from build123d import *

# Parameters (mm, degrees)
SKETCH3_W               = 1.778
SKETCH3_H               = 21.844
SKETCH4_W               = 63.2968
SKETCH4_H               = 43.561
BOSS_EXTRUDE1_DEPTH     = 1.778
BOSS_EXTRUDE2_DEPTH     = 1.778
SKETCH6_R               = 1.8034
BOSS_EXTRUDE3_DEPTH     = 5.08
FILLET2_R               = 3.81
SKETCH7_R               = 1.8034
BOSS_EXTRUDE4_DEPTH     = 25.4
CUT_EXTRUDE1_DEPTH      = 82.893164904
CUT_EXTRUDE1_DEPTH_BACK = 82.893164904
SKETCH8_W               = 7.5438
SKETCH8_H               = 10.541
SKETCH13_R              = 2.52476
BOSS_EXTRUDE5_DEPTH     = 63.2968
SKETCH14_W              = 27.40279
SKETCH14_H              = 7.62
SKETCH14_H_2            = 8.382
SKETCH14_W_2            = 3.45694
CUT_EXTRUDE2_DEPTH      = 80.858589657
FILLET3_R               = 8.382
FILLET4_R               = 1.27


# Some blends are built 0.0001 mm under size
with BuildPart() as part:
    # Sweep1: sweep along a path in Sketch1
    with BuildLine(Plane.XY) as sweep1_path:
        Line((0, 41.783), (0, 0))
        Line((0, 0), (59.7408, 0))
        Line((59.7408, 0), (59.7408, 41.783))
    # Sketch3 → Sweep1 (sweep)
    with BuildSketch(Plane(origin=(0, 41.783, 0), x_dir=(1, 0, 0), z_dir=(0, 1, 0))):
        with Locations((-0.889, 0)):
            Rectangle(SKETCH3_W, SKETCH3_H)
    sweep(path=sweep1_path.line, transition=Transition.RIGHT)

    # Sketch4 → Boss-Extrude1 (add)
    with BuildSketch(Plane(origin=(0, 0, -10.922), x_dir=(-1, 0, 0), z_dir=(0, 0, -1))):
        with Locations((-29.8704, 20.0025)):
            Rectangle(SKETCH4_W, SKETCH4_H)
    extrude(amount=BOSS_EXTRUDE1_DEPTH)

    # Sketch5 → Boss-Extrude2 (add)
    # profile 1 of 2: a face of its own
    with BuildSketch(Plane.XY.offset(10.922)):
        with BuildLine():
            Line((30.2514, 41.783), (0, 41.783))
            Line((0, 41.783), (0, 0))
            Line((0, 0), (59.7408, 0))
            Line((59.7408, 0), (59.7408, 41.783))
            Line((59.7408, 41.783), (58.20156, 41.783))
            Line((58.20156, 41.783), (58.20156, 27.91968))
            ThreePointArc((58.20156, 27.91968), (44.22648, 13.9446), (30.2514, 27.91968))
            Line((30.2514, 27.91968), (30.2514, 41.783))
        make_face()
        with BuildLine():
            Line((4.445, 5.4864), (4.445, 34.798))
            ThreePointArc((4.445, 34.798), (5.188948776, 36.594051224), (6.985, 37.338))
            Line((6.985, 37.338), (18.6182, 37.338))
            ThreePointArc((18.6182, 37.338), (20.414251224, 36.594051224), (21.1582, 34.798))
            Line((21.1582, 34.798), (21.1582, 24.296354404))
            ThreePointArc((21.1582, 24.296354404), (21.641564969, 21.866314608), (23.018071939, 19.806226343))
            Line((23.018071939, 19.806226343), (25.343528061, 17.480770222))
            ThreePointArc((25.343528061, 17.480770222), (26.720035031, 15.420681957), (27.2034, 12.990642162))
            Line((27.2034, 12.990642162), (27.2034, 5.4864))
            ThreePointArc((27.2034, 5.4864), (26.459451224, 3.690348776), (24.6634, 2.9464))
            Line((24.6634, 2.9464), (6.985, 2.9464))
            ThreePointArc((6.985, 2.9464), (5.188948776, 3.690348776), (4.445, 5.4864))
        make_face(mode=Mode.SUBTRACT)
    # profile 2 of 2: a face of its own
    with BuildSketch(Plane.XY.offset(10.922)):
        Polygon((61.5188, 41.783), (59.7408, 41.783), (59.7408, 0), (0, 0), (0, 41.783), (-1.778, 41.783), (-1.778, -1.778), (61.5188, -1.778), align=None)
    extrude(amount=BOSS_EXTRUDE2_DEPTH)

    # Sketch6 → Boss-Extrude3 (add)
    with BuildSketch(Plane(origin=(0, 41.783, 0), x_dir=(1, 0, 0), z_dir=(0, 1, 0))):
        with BuildLine():
            Line((64.5922, 3.5814), (61.5188, 3.5814))
            Line((61.5188, 3.5814), (61.5188, -3.5814))
            Line((61.5188, -3.5814), (64.5922, -3.5814))
            ThreePointArc((64.5922, -3.5814), (68.1736, 0), (64.5922, 3.5814))
        make_face()
        with Locations(Location((64.5922, 0, 0), (0, 0, 180))):
            Circle(SKETCH6_R, mode=Mode.SUBTRACT)
    extrude(amount=-BOSS_EXTRUDE3_DEPTH)

    # Fillet2
    # the kernel refuses this fillet: 3.81 mm, written as the material it adds along each edge
    with BuildSketch(Plane(origin=(61.5188, 41.783, -3.5814), x_dir=(0, 0, -1), z_dir=(0, -1, 0))) as fillet2_piece_1:
        with BuildLine():
            CenterArc((3.773204979, 3.81), FILLET2_R, 185.719382358, 84.280617642)
            Line((-0.017828515, 3.430309278), (-0.396931865, 3.392340206))
            ThreePointArc((-0.396931865, 3.392340206), (-0.381, 3.0734), (-0.381, 0))
            Line((-0.381, 0), (0, -0.381))
            Line((0, -0.381), (3.773204979, -0.381))
            Line((3.773204979, -0.381), (3.773204979, 0))
        make_face()
    extrude(amount=5.08)
    with BuildSketch(Plane(origin=(61.5188, 41.783, 3.5814), x_dir=(0, 0, 1), z_dir=(0, -1, 0))) as fillet2_piece_2:
        with BuildLine():
            CenterArc((3.773204979, -3.81), FILLET2_R, 90, 84.280617642)
            Line((-0.017828515, -3.430309278), (-0.396931865, -3.392340206))
            ThreePointArc((-0.396931865, -3.392340206), (-0.381, -3.0734), (-0.381, 0))
            Line((-0.381, 0), (0, 0.381))
            Line((0, 0.381), (3.773204979, 0.381))
            Line((3.773204979, 0.381), (3.773204979, 0))
        make_face()
    extrude(amount=5.08)

    # Sketch7 → Boss-Extrude4 (add)
    with BuildSketch(Plane.XY.offset(12.7)):
        with BuildLine():
            Line((-1.778, 36.3982), (-1.778, 41.783))
            Line((-1.778, 41.783), (-3.902308892, 43.053335031))
            ThreePointArc((-3.902308892, 43.053335031), (-8.404920605, 42.372664125), (-8.599730754, 37.82306259))
            Line((-8.599730754, 37.82306259), (-1.778, 28.7782))
            Line((-1.778, 28.7782), (-1.778, 36.3982))
        make_face()
        with Locations((-5.7404, 39.9796)):
            Circle(SKETCH7_R, mode=Mode.SUBTRACT)
    extrude(amount=-BOSS_EXTRUDE4_DEPTH)

    # Sketch8 → Cut-Extrude1 (cut, two sides: drawn at the far end of the back side and taken through both)
    with BuildSketch(Plane(origin=(0, 41.783, 0), x_dir=(1, 0, 0), z_dir=(0, 1, 0)).offset(-CUT_EXTRUDE1_DEPTH_BACK)):
        with Locations((-5.5499, 7.4295)):
            Rectangle(SKETCH8_W, SKETCH8_H)
        with Locations((-5.5499, -7.4295)):
            Rectangle(SKETCH8_W, SKETCH8_H)
    extrude(amount=CUT_EXTRUDE1_DEPTH + CUT_EXTRUDE1_DEPTH_BACK, mode=Mode.SUBTRACT)

    # Sketch13 → Boss-Extrude5 (add)
    with BuildSketch(Plane.ZY.offset(1.778)):
        with BuildLine():
            Line((-21.082, -1.778), (-12.7, -1.778))
            Line((-12.7, -1.778), (-12.7, 13.462))
            Line((-12.7, 13.462), (-21.082, 13.462))
            ThreePointArc((-21.082, 13.462), (-28.702, 5.842), (-21.082, -1.778))
        make_face()
        with Locations((-21.082, 5.842)):
            Circle(SKETCH13_R, mode=Mode.SUBTRACT)
    extrude(amount=-BOSS_EXTRUDE5_DEPTH)

    # Sketch14 → Cut-Extrude2 (cut, through all)
    with BuildSketch(Plane(origin=(0, 13.462, 0), x_dir=(1, 0, 0), z_dir=(0, 1, 0))):
        with Locations((11.923395, 24.892)):
            Rectangle(SKETCH14_W, SKETCH14_H)
        with Locations((11.923395, 16.891)):
            Rectangle(SKETCH14_W, SKETCH14_H_2)
        with Locations((47.817405, 16.891)):
            Rectangle(SKETCH14_W, SKETCH14_H_2)
        with Locations((47.817405, 24.892)):
            Rectangle(SKETCH14_W, SKETCH14_H)
        with Locations((29.8704, 24.892)):
            Rectangle(SKETCH14_W_2, SKETCH14_H)
        with Locations((29.8704, 16.891)):
            Rectangle(SKETCH14_W_2, SKETCH14_H_2)
    extrude(amount=-CUT_EXTRUDE2_DEPTH, mode=Mode.SUBTRACT)

    # Fillet3
    fillet3_edges = [part.edges().sort_by_distance(p)[0] for p in [
        (26.88336, 13.462, -12.7),
        (32.85744, 13.462, -12.7),
    ]]
    fillet(fillet3_edges, radius=FILLET3_R - 0.0001)  # a hair under: the kernel refuses the full size

    # Fillet4
    fillet4_edges = [part.edges().sort_by_distance(p)[0] for p in [
        (61.5188, -1.778, 0),
        (-1.778, 20.0025, 12.7),
        (-1.778, -1.778, 0),
        (-1.778, 20.0025, -12.7),
        (11.923395, -1.778, -12.7),
        (47.817405, -1.778, -12.7),
        (29.8704, -1.778, -12.7),
        (61.5188, 20.0025, -12.7),
        (29.8704, -1.778, 12.7),
        (61.5188, 20.0025, 12.7),
    ]]
    fillet(fillet4_edges, radius=FILLET4_R)


solid = part.part
The model under review builds one solid part; all positions refer to its coordinate system, in mm. A direction names the side the tool comes from. Coordinates: 2 decimals unless noted, no trailing zeros. Write each loop counter-clockwise with the first axis right and the second up, starting at its lowest first coordinate (ties: lowest second). Pieces come first, ordered by that corner, then holes. Notation, with made-up numbers: (20, 50) -> (28, 50) arc R18 ccw to (28, 55) -> close; hole circle Ø3 at (-3.75, 18.5). An arc over 180 degrees is marked (long way). Answer in a Markdown table with one row per item.
1. For faces 1 (the cylindrical face through (62.5, 39.3, 4.8)), 2 (the cylindrical face through (20.394, 36.614, 11.799)), 3 (the cylindrical face through (44.534, 13.948, 11.799)), 4 (the flat face through (27.9, 41.783, -11.2)), 5 (the flat face through (30, 21, -10.922)), list the 3-axis set-ups (+Z, -Z, +X, -X, +Y, -Y) from which the entire face can be reached by the end or side of a thin tool; tool diameter is ignored.
Answers below:
| item | result |
|---|---|
| face 1 | +Z, +X, +Y, -Y |
| face 2 | +Z |
| face 3 | +Z, +Y |
| face 4 | +Z, -Z, +X, +Y |
| face 5 | +Y |
2. Wall thickness on probe 1 along X at (y, z) = (28.5, -3); probe 2 along Z at (x, y) = (22, 40); probe 3 along Z at (x, y) = (35.5, 31.5): over which ranges is each line inside the solid? List them lowest first. Write a range as [from, to].
Answers below:
| item | result |
|---|---|
| probe 1 | x = [-1.78, 0], [59.74, 61.52] |
| probe 2 | z = [-12.7, -10.92], [10.92, 12.7] |
| probe 3 | z = [-12.7, -10.92] |
3. We need section B-B, the plane z = 0. State the section outline as (x, y) points.
Answers below:
| item | result |
|---|---|
| outline | (-8.6, 37.82) -> (-1.78, 28.78) -> (-1.78, -0.51) arc R1.27 ccw to (-0.51, -1.78) -> (60.25, -1.78) arc R1.27 ccw to (61.52, -0.51) -> (61.52, 36.7) -> (62.79, 36.7) -> (62.79, 41.78) -> (59.74, 41.78) -> (59.74, 0) -> (0, 0) -> (0, 41.78) -> (-1.78, 41.78) -> (-3.9, 43.05) arc R3.58 ccw to start; (66.4, 36.7) -> (68.17, 36.7) -> (68.17, 41.78) -> (66.4, 41.78) -> close; hole circle Ø3.61 at (-5.74, 39.98) |
4. Clearance check with flat-ended pins moving along their axes: pin 1 Ø5 at (y, z) = (10.5, -19) entering from -X; pin 2 Ø4 at (x, y) = (22.5, 19) entering from -Z; pin 3 Ø20.5 at (x, z) = (28, 2) entering from +Y. State where each tip first meets the part, or that it passes through.
Answers below:
| item | result |
|---|---|
| pin 1 | stops at x = 25.62 |
| pin 2 | stops at z = -12.7 |
| pin 3 | stops at y = 41.78 |
5. We need section C-C, the plane z = -16.5. State the section outline as (x, y) points, and give its area (3 significant figures).
Answers below:
| item | result |
|---|---|
| outline | (25.62, -1.78) -> (28.14, -1.78) -> (28.14, 14.83) -> (25.62, 14.83) -> close; (31.6, -1.78) -> (34.12, -1.78) -> (34.12, 14.83) -> (31.6, 14.83) -> close |
| area | 83.6 mm^2 |
6. Draft analysis for pull direction X (two halves, no side actions). For faces 6 (the flat face through (-1.778, 21, 0)), 7 (the flat face through (30.251, 35, 12)), 8 (the cylindrical face through (32.84, 7.97, -19.72)), state which applies: +X half, -X half, draft (parallel to the pull), parting line (faces both ways), or undercut.
Answers below:
| item | result |
|---|---|
| face 6 | -X half |
| face 7 | undercut |
| face 8 | draft |
7. We need section A-A, the plane x = 19.5. State the section outline as (y, z) points.
Answers below:
| item | result |
|---|---|
| outline | (-1.78, -11.43) arc R1.27 ccw to (-0.51, -12.7) -> (41.78, -12.7) -> (41.78, -10.92) -> (0, -10.92) -> (0, 10.92) -> (2.95, 10.92) -> (2.95, 12.7) -> (-0.51, 12.7) arc R1.27 ccw to (-1.78, 11.43) -> close; (37.18, 10.92) -> (41.78, 10.92) -> (41.78, 12.7) -> (37.18, 12.7) -> close |
8. We need section D-D, the plane y = 16. State the section outline as (x, z) points (3 decimals).
Answers below:
| item | result |
|---|---|
| outline | (-1.778, -11.43) arc R1.27 ccw to (-0.508, -12.7) -> (25.625, -12.7) -> (25.625, -15.073) -> (28.142, -15.073) -> (28.142, -12.7) -> (31.599, -12.7) -> (31.599, -15.073) -> (34.116, -15.073) -> (34.116, -12.7) -> (60.249, -12.7) arc R1.27 ccw to (61.519, -11.43) -> (61.519, 11.43) arc R1.27 ccw to (60.249, 12.7) -> (51.522, 12.7) -> (51.522, 10.922) -> (59.741, 10.922) -> (59.741, -10.922) -> (0, -10.922) -> (0, 10.922) -> (4.445, 10.922) -> (4.445, 12.7) -> (-0.508, 12.7) arc R1.27 ccw to (-1.778, 11.43) -> close; (26.445, 10.922) -> (36.931, 10.922) -> (36.931, 12.7) -> (26.445, 12.7) -> close |
